Autodesk Inventor part; units mm, degrees
ref_plane "YZ Plane" through (0, 0, 0) normal (1, 0, 0) x (0, 1, 0)
ref_plane "XZ Plane" through (0, 0, 0) normal (0, 1, 0) x (-1, 0, 0)
ref_plane "XY Plane" through (0, 0, 0) normal (0, 0, 1) x (1, 0, 0)
ref_plane "Work Plane1" through (0, 0, 2) normal (0, 0, 1) x (1, 0, 0)
sketch "Sketch1" plane through (0, 0, 2) normal (0, 0, 1) x (1, 0, 0)
  line L0 (-37.0712, 14) -> (-9.0712, 14) construction
  line L1 (-9.0712, 14) -> (-9.0712, -14) construction
  line L2 (-9.0712, -14) -> (-37.0712, -14) construction
  line L3 (-37.0712, -14) -> (-37.0712, 14) construction
  line L4 (-4.0712, -19) -> (-4.0712, 19)
  line L5 (-4.0712, 19) -> (-42.0712, 19)
  line L6 (-42.0712, 19) -> (-42.0712, -19)
  line L7 (-42.0712, -19) -> (-4.0712, -19)
  circle A0 centre (-23.0712, 0) radius 12.8
  point P0 (0, 0)
  dimension "d0" = 5
extrude "Extrusion1" add sketch "Sketch1" along normal blind 8 contours L7 L6 L5 L4 | A0
sketch "Sketch3" plane through (0, 0, 2) normal (0, 0, -1) x (-1, 0, 0)
  circle A0 centre (9.0712, -14) radius 1.45 construction
  circle A1 centre (9.0712, -14) radius 2.45
  circle A2 centre (37.0712, -14) radius 1.45
  circle A3 centre (37.0712, -14) radius 1.95
  point P0 (0, 0)
  dimension "d8" = 1
  dimension "d10" = 0.5
chamfer "Chamfer1" distance 3 angle 45 4 edges at (-42.0712, 19, 6) (-4.0712, 19, 6) (-4.0712, -19, 6) (-42.0712, -19, 6)
hole "Hole1" at (-37.0712, -14, 2) direction (0, 0, 1) diameter 4 depth 0.1 tip angle 100
sketch "Sketch4" plane through (-4.0712, -19, 2) normal (1, 0, 0) x (0, 0, -1)
  line L0 (2, 4.45) -> (6, 4.45)
  line L1 (2, 1.55) -> (6, 1.55)
  line L2 (0, 0) -> (0, 38)
  arc A0 (2, 19) -> (2, 19) centre (1.5, 4.4206) ccw
  line L3 (-1.7782, 5) -> (-0.1, 7)
  line L4 (-1.7782, 5) -> (-0.1, 3)
  line L5 (-0.1, 7) -> (0.6045, 7)
  line L6 (0.6045, 7) -> (0.6045, 3)
  line L7 (0.6045, 3) -> (-0.1, 3)
  line L8 (-0.1, 3) -> (-0.1, 7)
extrude "Extrusion4" cut sketch "Sketch4" against normal blind 8 contours L7 L8 L5 L2 | L2 L5 L6 L7 | L4 L3 L8
ref_plane "Arbeitsebene2" through (-23.0712, -12, 2) normal (1, 0, 0) x (0, 0, -1)
ref_plane "Arbeitsebene3" through (-39.0712, 0, 2) normal (0, -1, 0) x (1, 0, 0)
sketch "Skizze9" plane through (0, 0, 2) normal (0, 0, -1) x (-1, 0, 0)
  line L0 (12.0712, -16) -> (4.0712, -16)
  line L1 (7.0712, -19) -> (4.0712, -16)
  line L2 (39.0712, -19) -> (7.0712, -19)
  line L3 (42.0712, -16) -> (39.0712, -19)
  line L4 (42.0712, 16) -> (42.0712, -16)
  line L5 (39.0712, 19) -> (42.0712, 16)
  line L6 (7.0712, 19) -> (39.0712, 19)
  line L7 (4.0712, 16) -> (7.0712, 19)
  line L8 (4.0712, -12) -> (4.0712, 16)
  line L9 (4.0712, -12) -> (12.0712, -12)
  line L10 (12.0712, -12) -> (12.0712, -16)
  circle A0 centre (37.0712, -14) radius 2
  circle A1 centre (28.0712, -14) radius 3
  circle A2 centre (9.0712, 5) radius 3
  point P0 (0, 0)
  dimension "d54" = 6
  dimension "d55" = 6
  dimension "d56" = 14
  dimension "d57" = 5
  dimension "d58" = 5
  dimension "d59" = 14
extrude "Extrusion9" cut sketch "Skizze9" against normal blind 3 draft -2 contours A1 | A2
sketch "Skizze10" plane through (0, 0, 10) normal (0, 0, 1) x (1, 0, 0)
  circle A0 centre (-9.0712, 5) radius 4.05
  circle A1 centre (-28.0712, -14) radius 4.55
  circle A2 centre (-9.0712, 5) radius 4
  circle A3 centre (-28.0712, -14) radius 2.8952
  circle A4 centre (-28.0712, -14) radius 4
  point P0 (0, 0)
  dimension "d62" = 8
  dimension "d63" = 8
extrude "Extrusion10" cut sketch "Skizze10" against normal blind 7.5 contours A2 | A3 | A4
sketch "Skizze11" plane through (0, 0, 10) normal (0, 0, 1) x (1, 0, 0)
  circle A0 centre (-28.0712, -14) radius 4
  circle A1 centre (-9.0712, 5) radius 4
  line L0 (-39.0712, -19) -> (-42.0712, -16)
  line L1 (-39.0712, -19) -> (-7.0712, -19)
  line L2 (-4.0712, -16) -> (-7.0712, -19)
  line L3 (-4.0712, -16) -> (-4.0712, 16)
  line L4 (-7.0712, 19) -> (-4.0712, 16)
  line L5 (-7.0712, 19) -> (-39.0712, 19)
  line L6 (-42.0712, 16) -> (-39.0712, 19)
  line L7 (-42.0712, 16) -> (-42.0712, -16)
  circle A2 centre (-23.1616, 0) radius 12.8
  point P0 (0, 0)
  dimension "d66" = 25.6
extrude "Extrusion11" cut sketch "Skizze11" against normal blind 4 contours A2 A0 | A0 A2 A1 | A2 A1 picked at (-27.171, -11.4329) picked at (-11.706, 4.065)
equation "\"d54\" = d55"
equation "\"d59\" = d56"
properties part number "20_Cube_Insert_Kinematic_Thorlabs_1inch_pro_magnetic"
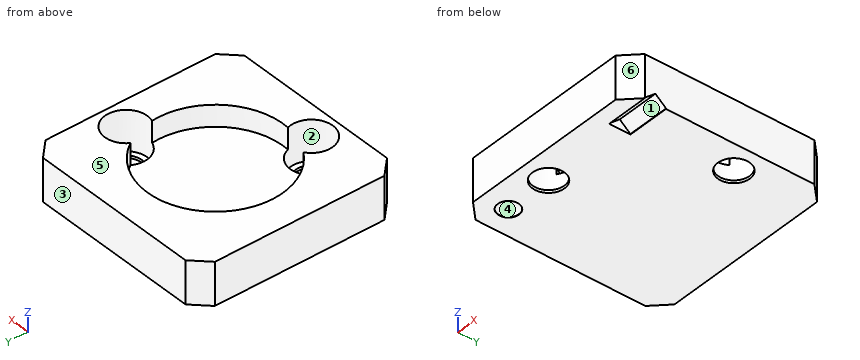
The listing builds one solid part. Answer for the finished solid, in the listing's coordinates (mm). Face numbers are marked on the shaded views. A direction names the side the tool comes from. Round coordinates to 2 decimals unless told otherwise and drop trailing zeros. Loops run counter-clockwise (first coordinate to the right, second up) from the corner with the lowest first, then second, coordinate; pieces in that order, holes last.
Q1. Given pin 1 Ø2.5 at (x, y) = (-26.5, -15.5) entering from +Z; pin 2 Ø7.5 at (x, y) = (-26.5, -3.5) entering from +Z; pin 3 Ø0.5 at (y, z) = (-15, 2.5) entering from +X, each flat-ended and moving along its own axis, determine where each tip first touches the part or whether it passes through.
Q2. Section C-C, the plane x = -20.5 is taken. Determine the outline of the cut face in (y, z), then the cut area to 3 significant figures.
Q3. Section A-A, the plane z = 4.25 is taken. Determine the outline of the cut face in (x, y), then the cut area to 3 significant figures.
Q4. Section D-D, the plane y = 5 is taken. Determine the outline of the cut face in (x, z).
Q5. Find the intervals of material crossed by line 1 (X direction, y = -14, z = 7.5); line 2 (Y direction, x = -13, z = 9); line 3 (Z direction, x = -18, y = -2), in increasing order.
Q6. Section B-B, the plane y = 0 is taken. Determine the outline of the cut face in (x, z), then the cut area to 3 significant figures.
Q7. Which of the six approach directions +Z, -Z, +X, -X, +Y, -Y give full straight-line access (tool end or side, diameter ignored) to the marked faces 1, 2 and 3?
Q8. For a pull along Y with two mould halves and no side action, classify the marked faces 4, 5 and 6 as released by +Y, released by -Y, zero draft, split by the parting line, or undercut.
Completed:
1. pin 1: stops at z = 2.5
1. pin 2: stops at z = 6
1. pin 3: stops at x = -12.07
2. outline: (-19, 2) - (19, 2) - (19, 10) - (12.52, 10) - (12.52, 6) - (-12.52, 6) - (-12.52, 10) - (-19, 10) - close
2. area: 204 mm2
3. outline: (-42.07, -16) - (-39.07, -19) - (-7.07, -19) - (-4.07, -16) - (-4.07, 16) - (-7.07, 19) - (-39.07, 19) - (-42.07, 16) - close; hole circle Ø8 at (-28.07, -14); hole circle Ø8 at (-9.07, 5)
3. area: 1,330 mm2
4. outline: (-42.07, 2) - (-12.07, 2) - (-12.05, 2.5) - (-13.07, 2.5) - (-13.07, 6) - (-34.94, 6) - (-34.94, 10) - (-42.07, 10) - close; (-6.09, 2.5) - (-6.07, 2) - (-4.07, 2) - (-4.07, 10) - (-5.07, 10) - (-5.07, 2.5) - close
5. line 1: x = -42.07 to -32.07, -24.07 to -4.07
5. line 2: y = -19 to -7.78, 7.78 to 19
5. line 3: z = 2 to 6
6. outline: (-42.07, 2) - (-4.07, 2) - (-4.07, 10) - (-10.36, 10) - (-10.36, 6) - (-35.96, 6) - (-35.96, 10) - (-42.07, 10) - close
6. area: 202 mm2
7. face 1: -Z, +X
7. face 2: +Z
7. face 3: +Z, -Z, +X, -X, +Y
8. face 4: undercut
8. face 5: zero draft
8. face 6: released by -Y
